Geometry check sheet. Reference: the model listing, model coordinates, mm. A direction names the side the tool comes from. Round coordinates to 2 decimals unless told otherwise and drop trailing zeros. Write each loop counter-clockwise with the first axis right and the second up, starting at its lowest first coordinate (ties: lowest second). Pieces come first, ordered by that corner, then holes. Notation, with made-up numbers: M 63.25,44 L 90.25,44 A24 ccw 90.25,71 Z; hole C 4,-25 d10. An arc over 180 degrees is marked long. Put each result on its own line as item: value. Start each with the question number.
(1) Material ranges on probe 1 along Z at (x, y) = (-105, 1.5); probe 2 along Y at (x, z) = (-76.2, -3); probe 3 along Y at (x, z) = (-76.2, -5), recorded low to high.
(2) Section check D-D on x = -121. Record the cut outline in (y, z), then the cut area to 3 significant figures.
(3) Gauge pin test, flat ends, axial feed: pin 1 (2.5 mm diameter, centred on x = -5.5, z = -3.5, fed in from +Y); pin 2 (1.4 mm diameter, centred on y = 5.5, z = -2, fed in from +X); pin 3 (3 mm diameter, centred on x = -89.5, z = -3, fed in from -Y). Record the tip position at first contact, or that the pin passes through.
(4) Mould release check, pull along Z, two halves, no side actions. Record for faces 1 (the flat face through (-77, 9, 0)), 2 (the flat face through (-77.3, 3.6, -6.35)), 3 (the cylindrical face through (-3.683, 6.367, -3.151)), 4 (the flat face through (-75.1, 9.3, -1.427)): pulls with the +Z half, pulls with the -Z half, needs draft (parallel to the pull), parting line crosses it, or undercut.
(5) Tool access check on faces 5 (the cylindrical face through (-148.716, 6.291, -3.151)), 6 (the flat face through (-6, 3.969, -3)), 7 (the flat face through (-75, 3.683, -3)), 8 (the flat face through (-75, 9.017, -3)). Record the directions out of +Z, -Z, +X, -X, +Y, -Y that give a thin tool (end or side, any length) a straight path to the whole face; none if there is none.
(6) Section check C-C on y = 10.5. Record the cut outline in (x, z), then the cut area to 3 significant figures.
(7) Section check A-A on z = -3.5. Record the cut outline in (x, y), then the cut area to 3 significant figures.
(8) Section check B-B on x = -76.2. Record the cut outline in (y, z).
from build123d import *

# Parameters (mm, degrees)
ESQUISSE1_W             = 152.4
ESQUISSE1_H             = 12.7
BOSS_EXTRU_1_DEPTH      = 6.35
ESQUISSE2_R             = 2.38125
ENL_V_MAT_EXTRU_1_DEPTH = 154.060029074
SKETCH1_W               = 14.17076538
SKETCH1_H               = 3.495000122
CUT_REVOLVE1_ANGLE      = 180
SKETCH2_W               = 3.495000122
SKETCH2_H               = 3.683
CUT_EXTRUDE1_DEPTH      = 154.060029074


with BuildPart() as part:
    # Esquisse1 → Boss.-Extru.1 (new body)
    with BuildSketch(Plane.XY):
        with Locations((-76.2, 6.35)):
            Rectangle(ESQUISSE1_W, ESQUISSE1_H)
    extrude(amount=-BOSS_EXTRU_1_DEPTH)

    # Esquisse2 → Enlèv. mat.-Extru.1 (cut, through all)
    with BuildSketch(Plane.XY):
        with Locations((-146.05, 6.35)):
            Circle(ESQUISSE2_R)
        with Locations((-76.2, 6.35)):
            Circle(ESQUISSE2_R)
        with Locations((-6.35, 6.35)):
            Circle(ESQUISSE2_R)
        with BuildLine():
            Line((0, 12.7), (-6.35, 12.7))
            ThreePointArc((-6.35, 12.7), (-1.859871939, 10.840128061), (0, 6.35))
            Line((0, 6.35), (0, 12.7))
        make_face()
        with BuildLine():
            Line((0, 0), (0, 6.35))
            ThreePointArc((0, 6.35), (-1.859871939, 1.859871939), (-6.35, 0))
            Line((-6.35, 0), (0, 0))
        make_face()
        with BuildLine():
            ThreePointArc((-152.4, 6.35), (-150.540128061, 10.840128061), (-146.05, 12.7))
            Line((-146.05, 12.7), (-152.4, 12.7))
            Line((-152.4, 12.7), (-152.4, 6.35))
        make_face()
        with BuildLine():
            ThreePointArc((-146.05, 0), (-150.540128061, 1.859871939), (-152.4, 6.35))
            Line((-152.4, 6.35), (-152.4, 0))
            Line((-152.4, 0), (-146.05, 0))
        make_face()
        with BuildLine():
            Line((-8.73125, 8.73125), (-8.73125, 6.35))
            ThreePointArc((-8.73125, 6.35), (-8.033798023, 8.033798023), (-6.35, 8.73125))
            Line((-6.35, 8.73125), (-8.73125, 8.73125))
        make_face()
        with BuildLine():
            ThreePointArc((-6.35, 8.73125), (-4.666201977, 8.033798023), (-3.96875, 6.35))
            Line((-3.96875, 6.35), (-3.96875, 8.73125))
            Line((-3.96875, 8.73125), (-6.35, 8.73125))
        make_face()
        with BuildLine():
            ThreePointArc((-3.96875, 6.35), (-4.666201977, 4.666201977), (-6.35, 3.96875))
            Line((-6.35, 3.96875), (-3.96875, 3.96875))
            Line((-3.96875, 3.96875), (-3.96875, 6.35))
        make_face()
        with BuildLine():
            Line((-8.73125, 6.35), (-8.73125, 3.96875))
            Line((-8.73125, 3.96875), (-6.35, 3.96875))
            ThreePointArc((-6.35, 3.96875), (-8.033798023, 4.666201977), (-8.73125, 6.35))
        make_face()
    extrude(amount=-ENL_V_MAT_EXTRU_1_DEPTH, mode=Mode.SUBTRACT)

    # Sketch1 → Cut-Revolve1 (revolve, symmetric, cut)
    with BuildSketch(Plane(origin=(0, 6.35, 0), x_dir=(1, 0, 0), z_dir=(0, 1, 0))) as cut_revolve1_sk:
        Polygon((-150.5585, 1.427499939), (-152.4, 1.427499939), (-152.4, 4.922500061), (-150.5585, 4.922500061), (-148.717, 4.922500061), (-148.717, 1.427499939), align=None)
        with Locations((-159.48538269, 3.175)):
            Rectangle(SKETCH1_W, SKETCH1_H)
    cut_revolve1 = revolve(axis=Axis((-146.05, 6.35, -6.35), (0, 0, 1)), revolution_arc=CUT_REVOLVE1_ANGLE / 2, mode=Mode.SUBTRACT)
    cut_revolve1 = cut_revolve1 + revolve(cut_revolve1_sk.sketch, axis=Axis((-146.05, 6.35, -6.35), (0, 0, -1)), revolution_arc=CUT_REVOLVE1_ANGLE / 2, mode=Mode.SUBTRACT)

    # Mirror1: Cut-Revolve1 across plane
    add(cut_revolve1.mirror(Plane(origin=(-76.2, 0, 0), x_dir=(0, 0, 1), z_dir=(1, 0, 0))), mode=Mode.SUBTRACT)

    # Sketch2 → Cut-Extrude1 (cut, through all)
    with BuildSketch(Plane(origin=(0, 0, 0), x_dir=(0, 0, -1), z_dir=(1, 0, 0))):
        with Locations((3.175, 10.8585)):
            Rectangle(SKETCH2_W, SKETCH2_H)
    cut_extrude1 = extrude(amount=-CUT_EXTRUDE1_DEPTH, mode=Mode.SUBTRACT)

    # Mirror2: Cut-Extrude1 across plane
    add(cut_extrude1.mirror(Plane.ZX.offset(6.35)), mode=Mode.SUBTRACT)


solid = part.part
Answers follow:
1. probe 1: z = -6.35 to -4.92, -1.43 to 0
1. probe 2: y = 3.68 to 3.97, 8.73 to 9.02
1. probe 3: y = 0 to 3.97, 8.73 to 12.7
2. outline: M 0,-6.35 L 12.7,-6.35 L 12.7,-4.92 L 9.02,-4.92 L 9.02,-1.43 L 12.7,-1.43 L 12.7,0 L 0,0 L 0,-1.43 L 3.68,-1.43 L 3.68,-4.92 L 0,-4.92 Z
2. area: 54.9 mm^2
3. pin 1: stops at y = 9.02
3. pin 2: stops at x = -0.02
3. pin 3: stops at y = 3.68
4. face 1: pulls with the +Z half
4. face 2: pulls with the -Z half
4. face 3: undercut
4. face 4: undercut
5. face 5: -X
5. face 6: +Z, -Z
5. face 7: +X, -X, -Y
5. face 8: +X, -X, +Y
6. outline: M -150.86,-6.35 L -1.54,-6.35 L -1.54,-4.92 L -150.86,-4.92 Z; M -150.86,-1.43 L -1.54,-1.43 L -1.54,0 L -150.86,0 Z
6. area: 426 mm^2
7. outline: M -146.05,3.68 L -6.35,3.68 A2.67 ccw -5.15,3.97 L -8.73,3.97 L -8.73,8.73 L -5.15,8.73 A2.67 ccw -6.35,9.02 L -146.05,9.02 A2.67 ccw Z; M -3.97,5.15 A2.67 ccw -3.97,7.55 Z; hole C -146.05,6.35 d4.76; hole C -76.2,6.35 d4.76
7. area: 710 mm^2
8. outline: M 0,-6.35 L 3.97,-6.35 L 3.97,0 L 0,0 L 0,-1.43 L 3.68,-1.43 L 3.68,-4.92 L 0,-4.92 Z; M 8.73,-6.35 L 12.7,-6.35 L 12.7,-4.92 L 9.02,-4.92 L 9.02,-1.43 L 12.7,-1.43 L 12.7,0 L 8.73,0 Z
